Design review of the part built by this model. Coordinates are the model's own, in mm. A direction names the side the tool comes from. Give positions to 0.01 mm unless a question says otherwise; leave off trailing zeros. Loops run counter-clockwise (first coordinate to the right, second up) from the corner with the lowest first, then second, coordinate; pieces in that order, holes last. Notation, with made-up numbers: (-4, -4.5) - (34, -4.5) arc R22 ccw to (34, 19.5) - close; hole circle Ø4 at (-31, 79). An arc over 180 degrees is marked (long way). Write each question's results on one line, items separated by ' | '.
```python
from build123d import *

# Parameters (mm, degrees)
SKETCH1_W               = 152.4
SKETCH1_H               = 12.7
BOSS_EXTRUDE1_DEPTH     = 76.2
SKETCH2_R               = 3.4925
BOSS_EXTRUDE4_DEPTH     = 3.175
BOSS_EXTRUDE5_DEPTH     = 12.7
CUT_EXTRUDE1_REACH      = 148.188
SKETCH4_R               = 3.4925
CUT_EXTRUDE2_DEPTH      = 147.187978302
CUT_EXTRUDE2_DEPTH_BACK = 147.187978302
SKETCH5_R               = 3.4925


with BuildPart() as part:
    # Sketch1 → Boss-Extrude1 (new body)
    with BuildSketch(Plane(origin=(0, 0, 0), x_dir=(1, 0, 0), z_dir=(0, 1, 0))):
        Rectangle(SKETCH1_W, SKETCH1_H)
    extrude(amount=BOSS_EXTRUDE1_DEPTH)

    # Sketch2 → Boss-Extrude4 (add)
    with BuildSketch(Plane(origin=(0, 0, 0), x_dir=(1, 0, 0), z_dir=(0, 1, 0))):
        Polygon((-76.2, 19.05), (-76.2, 6.35), (76.2, 6.35), (76.2, 31.75), (-76.2, 31.75), align=None)
        with Locations(Location((-63.5, 19.05, 0), (0, 0, 270))):
            Circle(SKETCH2_R, mode=Mode.SUBTRACT)
        with Locations(Location((-38.1, 19.05, 0), (0, 0, 270))):
            Circle(SKETCH2_R, mode=Mode.SUBTRACT)
        with Locations(Location((-12.7, 19.05, 0), (0, 0, 270))):
            Circle(SKETCH2_R, mode=Mode.SUBTRACT)
        with Locations(Location((12.7, 19.05, 0), (0, 0, 270))):
            Circle(SKETCH2_R, mode=Mode.SUBTRACT)
        with Locations(Location((38.1, 19.05, 0), (0, 0, 270))):
            Circle(SKETCH2_R, mode=Mode.SUBTRACT)
        with Locations(Location((63.5, 19.05, 0), (0, 0, 270))):
            Circle(SKETCH2_R, mode=Mode.SUBTRACT)
    extrude(amount=BOSS_EXTRUDE4_DEPTH)

    # Sketch3 → Boss-Extrude5 (add)
    with BuildSketch(Plane.XY.offset(6.35)):
        Polygon((-76.2, 76.2), (-76.2, 120.65), (76.2, 120.65), (76.2, 76.2), (73.025, 76.2), (73.025, 117.475), (-73.025, 117.475), (-73.025, 76.2), align=None)
    extrude(amount=-BOSS_EXTRUDE5_DEPTH)

    # Sketch4 → Cut-Extrude1 (cut, up to next)
    with BuildSketch(Plane(origin=(0, 120.65, 0), x_dir=(1, 0, 0), z_dir=(0, 1, 0)), mode=Mode.PRIVATE) as cut_extrude1_sk1:
        with Locations(Location((-25.4, 0, 0), (0, 0, 270))):
            Circle(SKETCH4_R)
    cut_extrude1_tool1 = extrude(cut_extrude1_sk1.sketch, amount=-CUT_EXTRUDE1_REACH, mode=Mode.PRIVATE) & part.part
    # Sketch4 → Cut-Extrude1 (cut, up to next)
    with BuildSketch(Plane(origin=(0, 120.65, 0), x_dir=(1, 0, 0), z_dir=(0, 1, 0)), mode=Mode.PRIVATE) as cut_extrude1_sk2:
        with Locations(Location((-16.256, 0, 0), (0, 0, 270))):
            Circle(SKETCH4_R)
    cut_extrude1_tool2 = extrude(cut_extrude1_sk2.sketch, amount=-CUT_EXTRUDE1_REACH, mode=Mode.PRIVATE) & part.part
    # Sketch4 → Cut-Extrude1 (cut, up to next)
    with BuildSketch(Plane(origin=(0, 120.65, 0), x_dir=(1, 0, 0), z_dir=(0, 1, 0)), mode=Mode.PRIVATE) as cut_extrude1_sk3:
        with Locations(Location((-7.112, 0, 0), (0, 0, 270))):
            Circle(SKETCH4_R)
    cut_extrude1_tool3 = extrude(cut_extrude1_sk3.sketch, amount=-CUT_EXTRUDE1_REACH, mode=Mode.PRIVATE) & part.part
    # Sketch4 → Cut-Extrude1 (cut, up to next)
    with BuildSketch(Plane(origin=(0, 120.65, 0), x_dir=(1, 0, 0), z_dir=(0, 1, 0)), mode=Mode.PRIVATE) as cut_extrude1_sk4:
        with Locations(Location((2.032, 0, 0), (0, 0, 270))):
            Circle(SKETCH4_R)
    cut_extrude1_tool4 = extrude(cut_extrude1_sk4.sketch, amount=-CUT_EXTRUDE1_REACH, mode=Mode.PRIVATE) & part.part
    # Sketch4 → Cut-Extrude1 (cut, up to next)
    with BuildSketch(Plane(origin=(0, 120.65, 0), x_dir=(1, 0, 0), z_dir=(0, 1, 0)), mode=Mode.PRIVATE) as cut_extrude1_sk5:
        with Locations(Location((11.176, 0, 0), (0, 0, 270))):
            Circle(SKETCH4_R)
    cut_extrude1_tool5 = extrude(cut_extrude1_sk5.sketch, amount=-CUT_EXTRUDE1_REACH, mode=Mode.PRIVATE) & part.part
    # Sketch4 → Cut-Extrude1 (cut, up to next)
    with BuildSketch(Plane(origin=(0, 120.65, 0), x_dir=(1, 0, 0), z_dir=(0, 1, 0)), mode=Mode.PRIVATE) as cut_extrude1_sk6:
        with Locations(Location((20.32, 0, 0), (0, 0, 270))):
            Circle(SKETCH4_R)
    cut_extrude1_tool6 = extrude(cut_extrude1_sk6.sketch, amount=-CUT_EXTRUDE1_REACH, mode=Mode.PRIVATE) & part.part
    # Sketch4 → Cut-Extrude1 (cut, up to next)
    with BuildSketch(Plane(origin=(0, 120.65, 0), x_dir=(1, 0, 0), z_dir=(0, 1, 0)), mode=Mode.PRIVATE) as cut_extrude1_sk7:
        with Locations(Location((29.464, 0, 0), (0, 0, 270))):
            Circle(SKETCH4_R)
    cut_extrude1_tool7 = extrude(cut_extrude1_sk7.sketch, amount=-CUT_EXTRUDE1_REACH, mode=Mode.PRIVATE) & part.part
    # Sketch4 → Cut-Extrude1 (cut, up to next)
    with BuildSketch(Plane(origin=(0, 120.65, 0), x_dir=(1, 0, 0), z_dir=(0, 1, 0)), mode=Mode.PRIVATE) as cut_extrude1_sk8:
        with Locations(Location((38.608, 0, 0), (0, 0, 270))):
            Circle(SKETCH4_R)
    cut_extrude1_tool8 = extrude(cut_extrude1_sk8.sketch, amount=-CUT_EXTRUDE1_REACH, mode=Mode.PRIVATE) & part.part
    add(cut_extrude1_tool1.solids().sort_by_distance((-25.4, 120.65, 0))[0], mode=Mode.SUBTRACT)
    add(cut_extrude1_tool2.solids().sort_by_distance((-16.256, 120.65, 0))[0], mode=Mode.SUBTRACT)
    add(cut_extrude1_tool3.solids().sort_by_distance((-7.112, 120.65, 0))[0], mode=Mode.SUBTRACT)
    add(cut_extrude1_tool4.solids().sort_by_distance((2.032, 120.65, 0))[0], mode=Mode.SUBTRACT)
    add(cut_extrude1_tool5.solids().sort_by_distance((11.176, 120.65, 0))[0], mode=Mode.SUBTRACT)
    add(cut_extrude1_tool6.solids().sort_by_distance((20.32, 120.65, 0))[0], mode=Mode.SUBTRACT)
    add(cut_extrude1_tool7.solids().sort_by_distance((29.464, 120.65, 0))[0], mode=Mode.SUBTRACT)
    add(cut_extrude1_tool8.solids().sort_by_distance((38.608, 120.65, 0))[0], mode=Mode.SUBTRACT)

    # Sketch5 → Cut-Extrude2 (cut, two sides: drawn at the far end of the back side and taken through both)
    with BuildSketch(Plane.XY.offset(-CUT_EXTRUDE2_DEPTH_BACK)):
        with Locations((-57.15, 25.4)):
            Circle(SKETCH5_R)
        with Locations((-19.05, 25.4)):
            Circle(SKETCH5_R)
        with Locations((19.05, 25.4)):
            Circle(SKETCH5_R)
        with Locations((57.15, 25.4)):
            Circle(SKETCH5_R)
    extrude(amount=CUT_EXTRUDE2_DEPTH + CUT_EXTRUDE2_DEPTH_BACK, mode=Mode.SUBTRACT)


solid = part.part
```
Item 1: We need section C-C on y = 25.4. Give the boundary of the cut face in (x, z).
Output values:
outline: (-76.2, -6.35) - (-60.64, -6.35) - (-60.64, 6.35) - (-76.2, 6.35) - close; (-53.66, -6.35) - (-22.54, -6.35) - (-22.54, 6.35) - (-53.66, 6.35) - close; (-15.56, -6.35) - (15.56, -6.35) - (15.56, 6.35) - (-15.56, 6.35) - close; (22.54, -6.35) - (53.66, -6.35) - (53.66, 6.35) - (22.54, 6.35) - close; (60.64, -6.35) - (76.2, -6.35) - (76.2, 6.35) - (60.64, 6.35) - close
Item 2: Clearance check with flat-ended pins moving along their axes: P1, Ø10, axis at x = -55.5, y = 36.5, coming from the -Z side; P2, Ø4, axis at x = -16.256, z = 0, coming from the +Y side; P3, Ø7.5, axis at x = -13.5, z = -18.5, coming from the +Y side (3 decimals). State where each tip first meets the part, or that it passes through.
Output values:
P1: stops at z = -6.35 | P2: stops at y = 76.2 | P3: stops at y = 3.175
Item 3: We need section A-A on x = -31. Give the boundary of the cut face in (y, z) (3 decimals), then the cut area to 3 significant figures.
Output values:
outline: (0, -31.75) - (3.175, -31.75) - (3.175, -6.35) - (76.2, -6.35) - (76.2, 6.35) - (0, 6.35) - close; (117.475, -6.35) - (120.65, -6.35) - (120.65, 6.35) - (117.475, 6.35) - close | area: 1,090 mm²
Item 4: Wall thickness on probe 1 along Y at (x, z) = (-51.5, -4) (3 decimals); probe 2 along X at (y, z) = (108.5, -2) (3 decimals); probe 3 along Z at (x, y) = (-38.5, 39): over which ranges is each line inside the solid? List them lowest first.
Output values:
probe 1: y = 0 to 76.2, 117.475 to 120.65 | probe 2: x = -76.2 to -73.025, 73.025 to 76.2 | probe 3: z = -6.35 to 6.35
Item 5: Draft analysis for pull direction Y (two halves, no side actions). For faces 1 (the face through (-73.025, 97, 0)), 2 (the face through (-1, 3.175, -19)), 3 (the face through (1, 50, -6.35)), 4 (the face through (1, 117.475, -4)), state which applies: +Y half, -Y half, draft (parallel to the pull), parting line (faces both ways), or undercut.
Output values:
face 1: undercut | face 2: +Y half | face 3: draft | face 4: undercut
Item 6: Tool access review of faces 5 (the face through (-66.91, 1.57, -19.81)), 6 (the face through (73.025, 97, 0)), 7 (the face through (14.64, 119.08, -0.45)): name each direction out of +Z, -Z, +X, -X, +Y, -Y from which nothing blocks a thin tool from reaching the whole face with its end or side.
Output values:
face 5: +Y, -Y | face 6: +Z, -Z | face 7: +Y
Item 7: We need section B-B on z = -19.05. Give the boundary of the cut face in (x, y) (1 decimal), then the cut area to 3 significant figures.
Output values:
outline: (-76.2, 0) - (-67, 0) - (-67, 3.2) - (-76.2, 3.2) - close; (-60, 0) - (-41.6, 0) - (-41.6, 3.2) - (-60, 3.2) - close; (-34.6, 0) - (-16.2, 0) - (-16.2, 3.2) - (-34.6, 3.2) - close; (-9.2, 0) - (9.2, 0) - (9.2, 3.2) - (-9.2, 3.2) - close; (16.2, 0) - (34.6, 0) - (34.6, 3.2) - (16.2, 3.2) - close; (41.6, 0) - (60, 0) - (60, 3.2) - (41.6, 3.2) - close; (67, 0) - (76.2, 0) - (76.2, 3.2) - (67, 3.2) - close | area: 351 mm²
Item 8: We need section D-D on x = 57.15. Give the number of separate pieces and of enclosed holes in the cut face, then the cut area to 4 significant figures.
Output values:
separate pieces: 3 | enclosed holes: 0 | area: 1,000 mm²
